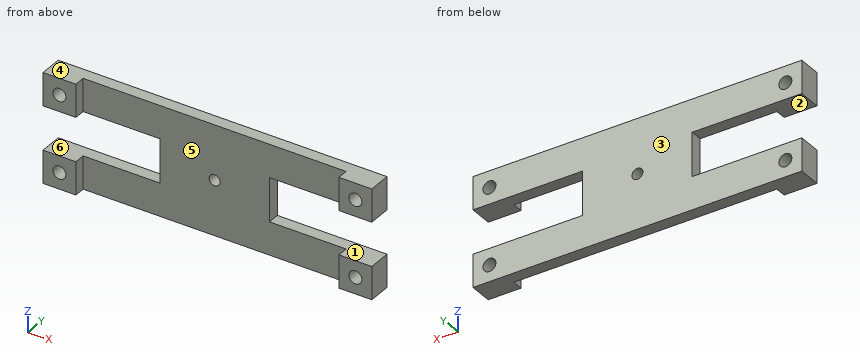
Autodesk Inventor part; units mm, degrees
ref_plane "YZ Plane" through (0, 0, 0) normal (1, 0, 0) x (0, 1, 0)
ref_plane "XZ Plane" through (0, 0, 0) normal (0, 1, 0) x (-1, 0, 0)
ref_plane "XY Plane" through (0, 0, 0) normal (0, 0, 1) x (1, 0, 0)
sketch "Sketch1" plane through (0, 0, 0) normal (0, 1, 0) x (-1, 0, 0)
  line L0 (8.5745, -14.965) -> (8.5745, 10.435)
  line L1 (8.5745, 10.435) -> (-16.8255, 10.435)
  line L2 (-16.8255, 10.435) -> (-16.8255, -14.965)
  line L3 (-16.8255, -14.965) -> (8.5745, -14.965)
  point P0 (0, 0)
  dimension "d0" = 25.4
  dimension "d1" = 25.4
extrude "Extrusion1" add sketch "Sketch1" along normal blind 2.794
sketch "Sketch2" plane through (16.8255, 0, 10.435) normal (1, 0, 0) x (0, 0, -1)
  line L0 (25.4, 2.794) -> (0, 2.794)
  line L1 (25.4, 0) -> (0, 0)
  line L2 (0, 2.794) -> (7.62, 2.794)
  line L3 (7.62, 2.794) -> (7.62, 0)
  line L4 (7.62, 0) -> (0, 0)
  line L5 (0, 0) -> (0, 2.794)
  line L6 (25.4, 0) -> (17.78, 0)
  line L7 (17.78, 0) -> (17.78, 2.794)
  line L8 (17.78, 2.794) -> (25.4, 2.794)
  line L9 (25.4, 2.794) -> (25.4, 0)
  point P0 (10.435, 0)
  dimension "d4" = 7.62
  dimension "d5" = 7.62
extrude "Extrusion2" add sketch "Sketch2" along normal blind 25.4 and the other way blind 50.8 contours L9 L1 L7 L0 | L3 L1 L5 L0
sketch "Sketch3" plane through (0, 0, 0) normal (0, -1, 0) x (1, 0, 0)
  line L0 (16.8255, 2.815) -> (16.8255, -7.345) construction
  line L1 (16.8255, -2.265) -> (-8.5745, -2.265) construction
  line L2 (-8.5745, -7.345) -> (-8.5745, 2.815) construction
  line L3 (42.2255, -14.965) -> (-33.9745, -14.965) construction
  line L4 (4.1255, -14.965) -> (4.1255, 10.435) construction
  line L5 (-33.9745, 10.435) -> (42.2255, 10.435) construction
  circle A0 centre (4.1255, -2.265) radius 1.27
  point P0 (0, 0)
  dimension "d10" = 2.54
extrude "Extrusion3" cut sketch "Sketch3" against normal blind 25.4
sketch "Sketch4" plane through (0, 0, 0) normal (0, -1, 0) x (1, 0, 0)
  line L0 (-33.9745, -14.965) -> (42.2255, -14.965)
  line L1 (16.8255, -7.345) -> (42.2255, -7.345)
  line L2 (42.2255, -14.965) -> (34.6055, -14.965)
  line L3 (34.6055, -14.965) -> (34.6055, -7.345)
  line L4 (34.6055, -7.345) -> (42.2255, -7.345)
  line L5 (42.2255, -7.345) -> (42.2255, -14.965)
  line L6 (42.2255, 10.435) -> (-33.9745, 10.435)
  line L7 (-33.9745, -7.345) -> (-33.9745, -14.965)
  line L8 (-33.9745, -7.345) -> (-8.5745, -7.345)
  line L9 (-33.9745, -14.965) -> (-26.3545, -14.965)
  line L10 (-26.3545, -14.965) -> (-26.3545, -7.345)
  line L11 (-26.3545, -7.345) -> (-33.9745, -7.345)
  line L12 (-33.9745, -7.345) -> (-33.9745, -14.965)
  line L13 (-33.9745, 10.435) -> (-33.9745, 2.815)
  line L14 (-33.9745, 2.815) -> (-26.3545, 2.815)
  line L15 (-26.3545, 2.815) -> (-26.3545, 10.435)
  line L16 (-26.3545, 10.435) -> (-33.9745, 10.435)
  line L17 (-33.9745, 10.435) -> (-33.9745, 2.815)
  line L18 (42.2255, 2.815) -> (42.2255, 10.435)
  line L19 (-33.9745, 10.435) -> (42.2255, 10.435)
  line L20 (42.2255, 2.815) -> (34.6055, 2.815)
  line L21 (34.6055, 2.815) -> (34.6055, 10.435)
  line L22 (34.6055, 10.435) -> (42.2255, 10.435)
  line L23 (42.2255, 10.435) -> (42.2255, 2.815)
  point P0 (0, 0)
  dimension "d13" = 7.62
  dimension "d14" = 7.62
  dimension "d15" = 7.62
extrude "Extrusion4" add sketch "Sketch4" along normal blind 2.54
sketch "Sketch5" plane through (0, -2.54, 0) normal (0, -1, 0) x (1, 0, 0)
  line L0 (42.2255, -14.965) -> (42.2255, -7.345)
  line L1 (34.6055, -14.965) -> (34.6055, -7.345)
  line L2 (42.2255, -14.965) -> (34.6055, -14.965)
  line L3 (34.6055, -14.965) -> (34.6055, -7.345)
  line L4 (34.6055, -7.345) -> (42.2255, -7.345)
  line L5 (42.2255, -7.345) -> (42.2255, -14.965)
  circle A0 centre (38.4155, -11.155) radius 1.5
  circle A1 centre (38.4155, 6.625) radius 1.5012
  line L6 (34.6055, 10.435) -> (34.6055, 2.815)
  circle A2 centre (-30.1645, 6.625) radius 1.5
  line L7 (-33.9745, 2.815) -> (-26.3545, 2.815)
  circle A3 centre (-30.1645, -11.155) radius 1.5
  point P0 (0, 0)
  point P1 (34.6055, 6.625)
  point P2 (-30.1645, 2.815)
  dimension "d18" = 3
  dimension "d19" = 3
  dimension "d20" = 3.0024
  dimension "d21" = 3
extrude "Extrusion5" cut sketch "Sketch5" against normal blind 76.2 contours A0 | A1 | A2 | A3
equation "\"d5\" = d4"
properties part number "Camera Mount"
CAD build for the part. Positions are in the model's coordinates, mm. Face numbers are marked on the shaded views. A direction names the side the tool comes from. Give positions to 0.01 mm unless a question says otherwise; leave off trailing zeros. Write each loop counter-clockwise with the first axis right and the second up, starting at its lowest first coordinate (ties: lowest second). Pieces come first, ordered by that corner, then holes. Notation, with made-up numbers: (11.25, 89.25) - (27.25, 89.25) arc R12 ccw to (27.25, 100.25) - close; hole circle Ø1 at (-6.5, 64.5). An arc over 180 degrees is marked (long way). Answer as CSV lines item,"result".
Q1. Drill centre lines: line 1 (Z direction, x = 21, y = 2) (3 decimals); line 2 (X direction, y = 1.45, z = 7); line 3 (X direction, y = -2.3, z = 5.5). Where is each one in solid material? Low to high. Write a range as from..to.
Result set:
line 1,"-14.965..-7.345, 2.815..10.435"
line 2,"-33.97..-31.62, -28.71..36.96, 39.87..42.23"
line 3,"-33.97..-31.16, -29.17..-26.35, 34.61..37.42, 39.41..42.23"
Q2. 3-axis set-ups, long thin cutter, end or side, ignore diameter. For the marked faces 1, 2 and 3: which of +Z, -Z, +X, -X, +Y, -Y reach the whole face in a straight line?
Result set:
face 1,"+X, +Y, -Y"
face 2,"-X, +Y, -Y"
face 3,"+Z, -Z, +X, -X, +Y"
Q3. Flat gauge pins, fed straight in: pin 1 Ø4 at (x, z) = (38.42, -11.16) entering from +Y; pin 2 Ø3 at (y, z) = (1, -3) entering from -X; pin 3 Ø2 at (y, z) = (2, -3) entering from +X. Where does each tip first touch, or does it go through?
Result set:
pin 1,"y = 2.79"
pin 2,"x = -8.57"
pin 3,"x = 16.83"
Q4. Band-saw the part on C-C (z = 4). Give the cut face in (x, y), and give its area (3 significant figures).
Result set:
outline,"(-33.97, -2.54) - (-26.35, -2.54) - (-26.35, 0) - (34.61, 0) - (34.61, -2.54) - (42.23, -2.54) - (42.23, 2.79) - (-33.97, 2.79) - close"
area,"252 mm²"
Q5. Band-saw the part on A-A (x = 19.5). Give the cut face in (y, z) (3 decimals).
Result set:
outline,"(0, -14.965) - (2.794, -14.965) - (2.794, -7.345) - (0, -7.345) - close; (0, 2.815) - (2.794, 2.815) - (2.794, 10.435) - (0, 10.435) - close"
Q6. Band-saw the part on B-B (y = -1). Give the cut face in (x, z) (1 decimal), and give its area (3 significant figures).
Result set:
outline,"(-34, -15) - (-26.4, -15) - (-26.4, -7.3) - (-34, -7.3) - close; (-34, 2.8) - (-26.4, 2.8) - (-26.4, 10.4) - (-34, 10.4) - close; (34.6, -15) - (42.2, -15) - (42.2, -7.3) - (34.6, -7.3) - close; (34.6, 2.8) - (42.2, 2.8) - (42.2, 10.4) - (34.6, 10.4) - close; hole circle Ø3 at (-30.2, -11.2); hole circle Ø3 at (-30.2, 6.6); hole circle Ø3 at (38.4, -11.2); hole circle Ø3 at (38.4, 6.6)"
area,"204 mm²"
Q7. Pull direction Z, two halves, no side cores. Call the marked faces 4, 5 and 6: released by +Z, released by -Z, zero draft, split by the parting line, or undercut.
Result set:
face 4,"released by +Z"
face 5,"zero draft"
face 6,"undercut"
Q8. Band-saw the part on D-D (x = 8.5). Give the cut face in (y, z) (3 decimals).
Result set:
outline,"(0, -14.965) - (2.794, -14.965) - (2.794, 10.435) - (0, 10.435) - close"
